The listing builds one solid part. Answer for the finished solid, in the listing's coordinates (mm). Face numbers are marked on the shaded views. Round coordinates to 2 decimals unless told otherwise and drop trailing zeros. Order: outer loops, then holes, each group sorted by start corner. A loop starts at its lowest first (then second) coordinate and runs counter-clockwise, first axis right, second up. Notation, with made-up numbers: (-12, -12.5) - (10, -12.5) arc R31 ccw to (10, 14.5) - close; hole circle Ø1 at (77.5, -40). An arc over 180 degrees is marked (long way). Use CSV: the item, a comma, the result in double quotes. Start each with the question number.
Item 1: Find section A-A, the plane z = 0.95. Give the vertices of the cut face in (x, y).
Item 2: Determine the mould class of the marked faces 1, 2 and 3 for opening direction Y: +Y half, -Y half, draft (parallel to the pull), parting line (faces both ways), or undercut.
Item 3: Find section D-D, the plane x = -8.25. Give the vertices of the cut face in (y, z), plus the area to 3 significant figures.
Item 4: Find section C-C, the plane y = 3.2. Give the vertices of the cut face in (x, z).
Item 5: Find section B-B, the plane x = 8.5. Give the vertices of the cut face in (y, z), plus the area to 3 significant figures.
Item 6: Straight lines are drawn through the part: line 1 along Y through (x, z) = (-9.25, 0.6); line 2 along X through (y, z) = (2.5, 0.85); line 3 along X through (y, z) = (1.7, 0.8). For each, find the intervals that lie inside material, in ascending order. Write a range as [from, to].
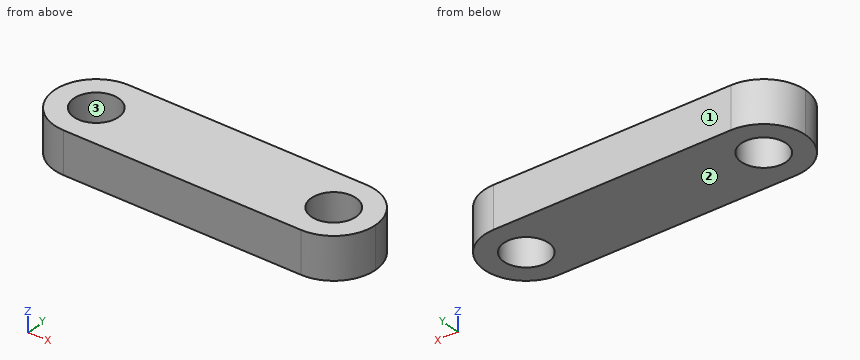
```python
from build123d import *

# Parameters (mm, degrees)
SKETCH_1_R          = 1.35
EXTRUDE_1_DEPTH     = 3
SKETCH_2_R          = 1.6
CUT_EXTRUDE_1_DEPTH = 14.922339711


with BuildPart() as part:
    # 草图1 → 凸台-拉伸1 (new body)
    with BuildSketch(Plane.XY.offset(3)):
        with BuildLine():
            Line((7.774087989, 5.999), (-9.200145164, 5.999))
            ThreePointArc((-9.200145164, 5.999), (-11.321465508, 5.120320344), (-12.200145164, 2.999))
            ThreePointArc((-12.200145164, 2.999), (-11.321112092, 0.878326133), (-9.200145331, 0))
            Line((-9.200145331, 0), (7.774087823, 0))
            ThreePointArc((7.774087823, 0), (9.895408166, 0.878679656), (10.774087823, 3))
            ThreePointArc((10.774087823, 3), (9.89505475, 5.120673867), (7.774087989, 5.999))
        make_face()
        with Locations((7.774087823, 3)):
            Circle(SKETCH_1_R, mode=Mode.SUBTRACT)
        with Locations((-9.200145331, 3)):
            Circle(SKETCH_1_R, mode=Mode.SUBTRACT)
    extrude(amount=-EXTRUDE_1_DEPTH)

    # 草图2 → 切除-拉伸1 (cut, through all)
    with BuildSketch(Plane.XY.offset(3)):
        with Locations((-9.200145331, 3)):
            Circle(SKETCH_2_R)
        with Locations((7.774087989, 2.999)):
            Circle(SKETCH_2_R)
    extrude(amount=-CUT_EXTRUDE_1_DEPTH, mode=Mode.SUBTRACT)


solid = part.part
```
Worked out:
1,outline,"(-12.2, 3) arc R3 ccw to (-9.2, 0) - (7.77, 0) arc R3 ccw to (10.77, 3) arc R3 ccw to (7.77, 6) - (-9.2, 6) arc R3 ccw to start; hole circle Ø3.2 at (-9.2, 3); hole circle Ø3.2 at (7.77, 3)"
2,face 1,"+Y half"
2,face 2,"draft"
2,face 3,"undercut"
3,outline,"(0, 0) - (1.71, 0) - (1.71, 3) - (0, 3) - close; (4.29, 0) - (6, 0) - (6, 3) - (4.29, 3) - close"
3,area,"10.3 mm²"
4,outline,"(-12.19, 0) - (-10.79, 0) - (-10.79, 3) - (-12.19, 3) - close; (-7.61, 0) - (6.19, 0) - (6.19, 3) - (-7.61, 3) - close; (9.36, 0) - (10.77, 0) - (10.77, 3) - (9.36, 3) - close"
5,outline,"(0.09, 0) - (1.57, 0) - (1.57, 3) - (0.09, 3) - close; (4.42, 0) - (5.91, 0) - (5.91, 3) - (4.42, 3) - close"
5,area,"8.91 mm²"
6,line 1,"y = [0, 1.4], [4.6, 6]"
6,line 2,"x = [-12.16, -10.72], [-7.68, 6.25], [9.29, 10.73]"
6,line 3,"x = [-11.9, -10.13], [-8.27, 6.84], [8.71, 10.48]"
